Verification items for the finished model (mm, model axes). Round coordinates to 2 decimals unless told otherwise and drop trailing zeros. Order: outer loops, then holes, each group sorted by start corner. A loop starts at its lowest first (then second) coordinate and runs counter-clockwise, first axis right, second up. Notation, with made-up numbers: (32.25, -21.5) -> (82.25, -21.5) arc R23 ccw to (82.25, 15.5) -> close; hole circle Ø3 at (-9.75, -24.75). An arc over 180 degrees is marked (long way). Write item = value, one per line. Start each with the question number.
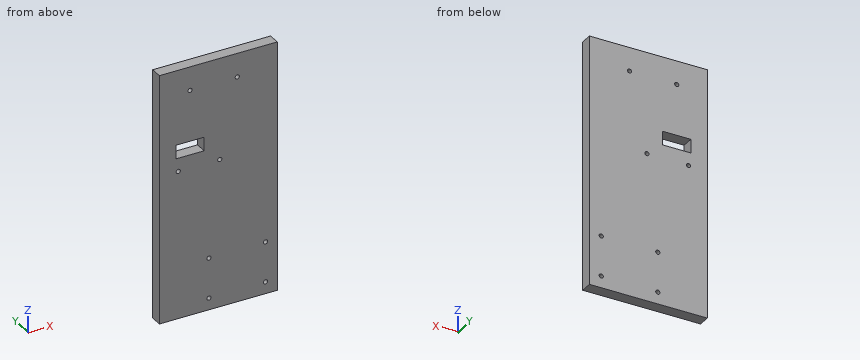
from build123d import *

# Parameters (mm, degrees)
SKETCH1_W             = 63.5
SKETCH1_H             = 134.112
BOSS_EXTRUDE1_DEPTH   = 6.35
SKETCH4_W             = 15.24
SKETCH4_H             = 7.366
CUT_EXTRUDE3_DEPTH    = 7.35
F_4_40_TAPPED_HOLE1_D = 2.2606
F_4_40_TAPPED_HOLE2_D = 2.2606
F_4_40_TAPPED_HOLE3_D = 2.2606


with BuildPart() as part:
    # Sketch1 → Boss-Extrude1 (new body)
    with BuildSketch(Plane(origin=(0, 0, 0), x_dir=(1, 0, 0), z_dir=(0, 1, 0))):
        with Locations((31.75, 67.056)):
            Rectangle(SKETCH1_W, SKETCH1_H)
    extrude(amount=BOSS_EXTRUDE1_DEPTH)

    # Sketch4 → Cut-Extrude3 (cut, through all)
    with BuildSketch(Plane(origin=(0, 6.35, 0), x_dir=(1, 0, 0), z_dir=(0, 1, 0))):
        with Locations((16.51, 43.815)):
            Rectangle(SKETCH4_W, SKETCH4_H)
    extrude(amount=-CUT_EXTRUDE3_DEPTH, mode=Mode.SUBTRACT)

    # #4-40 Tapped Hole1 (through all)
    with Locations(Plane(origin=(0, 6.35, 0), x_dir=(1, 0, 0), z_dir=(0, 1, 0))):
        with Locations((57.15, 127.762), (57.15, 106.172), (26.67, 106.172), (26.67, 127.762)):
            Hole(F_4_40_TAPPED_HOLE1_D / 2)

    # #4-40 Tapped Hole2 (through all)
    with Locations(Plane(origin=(0, 6.35, 0), x_dir=(1, 0, 0), z_dir=(0, 1, 0))):
        with Locations((32.512, 54.61), (10.16, 54.61)):
            Hole(F_4_40_TAPPED_HOLE2_D / 2)

    # #4-40 Tapped Hole3 (through all)
    with Locations(Plane(origin=(0, 6.35, 0), x_dir=(1, 0, 0), z_dir=(0, 1, 0))):
        with Locations((41.91, 12.7), (16.51, 12.7)):
            Hole(F_4_40_TAPPED_HOLE3_D / 2)


solid = part.part
(1) Cross-section at A-A (x = 14). Enter the section's corners in (y, z).
(2) Scan lines: line 1 along X through (y, z) = (3, -54.61); line 2 along Z through (x, y) = (57.15, 2.5); line 3 along X through (y, z) = (1.5, -12.7). Record each from-to range of solid material in increasing order. Write a range as from..to.
(3) Cross-section at B-B (z = -43.5). Enter the section's corners in (x, y), and give its area (3 significant figures).
(4) Cross-section at C-C (y = 2). Give the number of separate pieces and of enclosed holes in the cut face, and give its area (3 significant figures).
(5) Depth check by flat-ended pin: pin 1 (1 mm diameter, centred on x = 46, z = -17.5, fed in from -Y). Enter the tip coordinate at first touch or a pass-through.
Outcome:
q1.outline = (0, -134.11) -> (6.35, -134.11) -> (6.35, -47.5) -> (0, -47.5) -> close; (0, -40.13) -> (6.35, -40.13) -> (6.35, 0) -> (0, 0) -> close
q2.line_1 = 0..9.03, 11.29..31.38, 33.64..63.5
q2.line_2 = -134.11..-128.89, -126.63..-107.3, -105.04..0
q2.line_3 = 0..15.38, 17.64..40.78, 43.04..63.5
q3.outline = (0, 0) -> (8.89, 0) -> (8.89, 6.35) -> (0, 6.35) -> close; (24.13, 0) -> (63.5, 0) -> (63.5, 6.35) -> (24.13, 6.35) -> close
q3.area = 306 mm^2
q4.separate_pieces = 1
q4.enclosed_holes = 9
q4.area = 8,370 mm^2
q5.pin_1 = 0
